Design review of the part shown in the three views and the two pictorial views. Dimensions are in mm from the part's minimum x, y and z. A direction names the side the tool comes from. Give positions to 0.01 mm unless a question says otherwise; leave off trailing zeros. Loops run counter-clockwise (first coordinate to the right, second up) from the corner with the lowest first, then second, coordinate; pieces in that order, holes last. Notation, with made-up numbers: (-12, 70.5) - (44, 70.5) arc R33 ccw to (44, 106.5) - close; hole circle Ø4 at (61, 19). An arc over 180 degrees is marked (long way). Use CSV: the item, a comma, the result in double quotes. Start each with the question number.
1. Take a section at C-C on z = 10. Give the boundary of the cut face in (x, y).
2. For pin 1 (3 mm diameter, centred on x = 28.5, y = 9, fed in from -Z); pin 2 (3 mm diameter, centred on x = 20.5, y = 10.5, fed in from +Z), all flat-tipped, find the tip position at first contact; note any pin that passes through.
3. For the marked faces 1, 2 and 3, list the 3-axis set-ups (+Z, -Z, +X, -X, +Y, -Y) from which the entire face can be reached by the end or side of a thin tool; tool diameter is ignored.
4. Wall thickness on line 1 (Y direction, x = 55.5, z = 15); line 2 (Z direction, x = 49, y = 10); line 3 (Y direction, x = 50.5, z = 9.75): over which ranges is each line inside the solid? List them lowest first.
5. Take a section at A-A on x = 6.5. Give the boundary of the cut face in (y, z).
6. Take a section at B-B on y = 4.5. Give the boundary of the cut face in (x, z), plus the area to 3 significant figures.
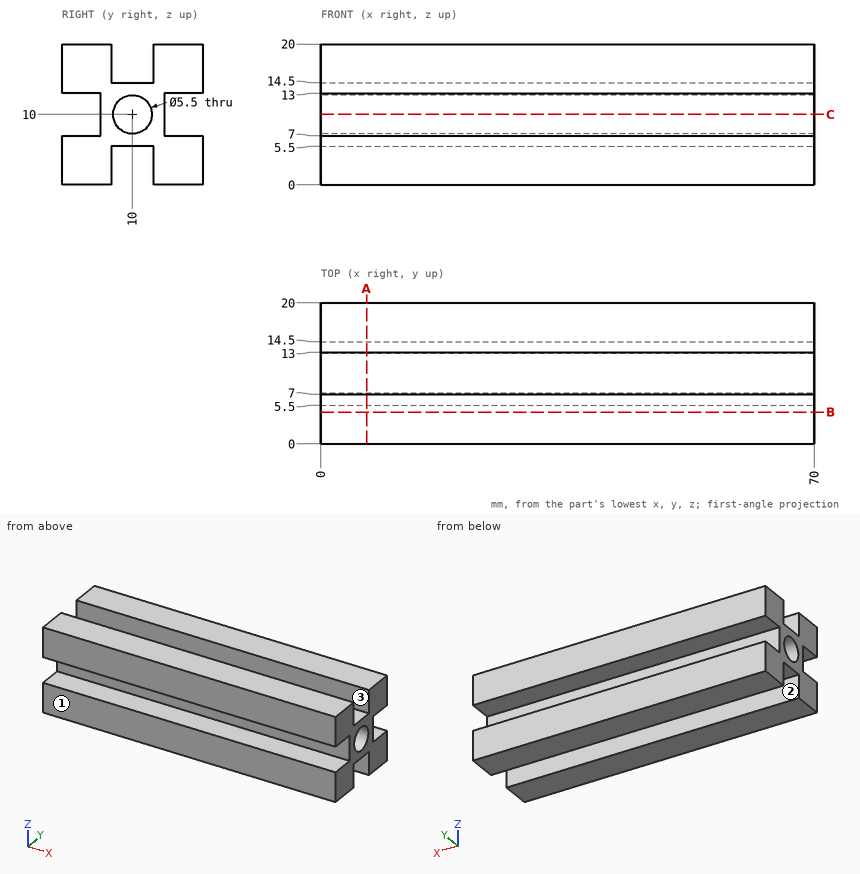
Check result:
1,outline,"(0, 5.5) - (70, 5.5) - (70, 7.25) - (0, 7.25) - close; (0, 12.75) - (70, 12.75) - (70, 14.5) - (0, 14.5) - close"
2,pin 1,"stops at z = 5.5"
2,pin 2,"stops at z = 14.5"
3,face 1,"+Z, -Z, +X, -X, -Y"
3,face 2,"-Z, +X, -X"
3,face 3,"+Z, +X, -X"
4,line 1,"y = 0 to 7, 13 to 20"
4,line 2,"z = 5.5 to 7.25, 12.75 to 14.5"
4,line 3,"y = 5.5 to 7.26, 12.74 to 14.5"
5,outline,"(0, 0) - (7, 0) - (7, 5.5) - (13, 5.5) - (13, 0) - (20, 0) - (20, 7) - (14.5, 7) - (14.5, 13) - (20, 13) - (20, 20) - (13, 20) - (13, 14.5) - (7, 14.5) - (7, 20) - (0, 20) - (0, 13) - (5.5, 13) - (5.5, 7) - (0, 7) - close; hole circle Ø5.5 at (10, 10)"
6,outline,"(0, 0) - (70, 0) - (70, 7) - (0, 7) - close; (0, 13) - (70, 13) - (70, 20) - (0, 20) - close"
6,area,"980 mm²"
